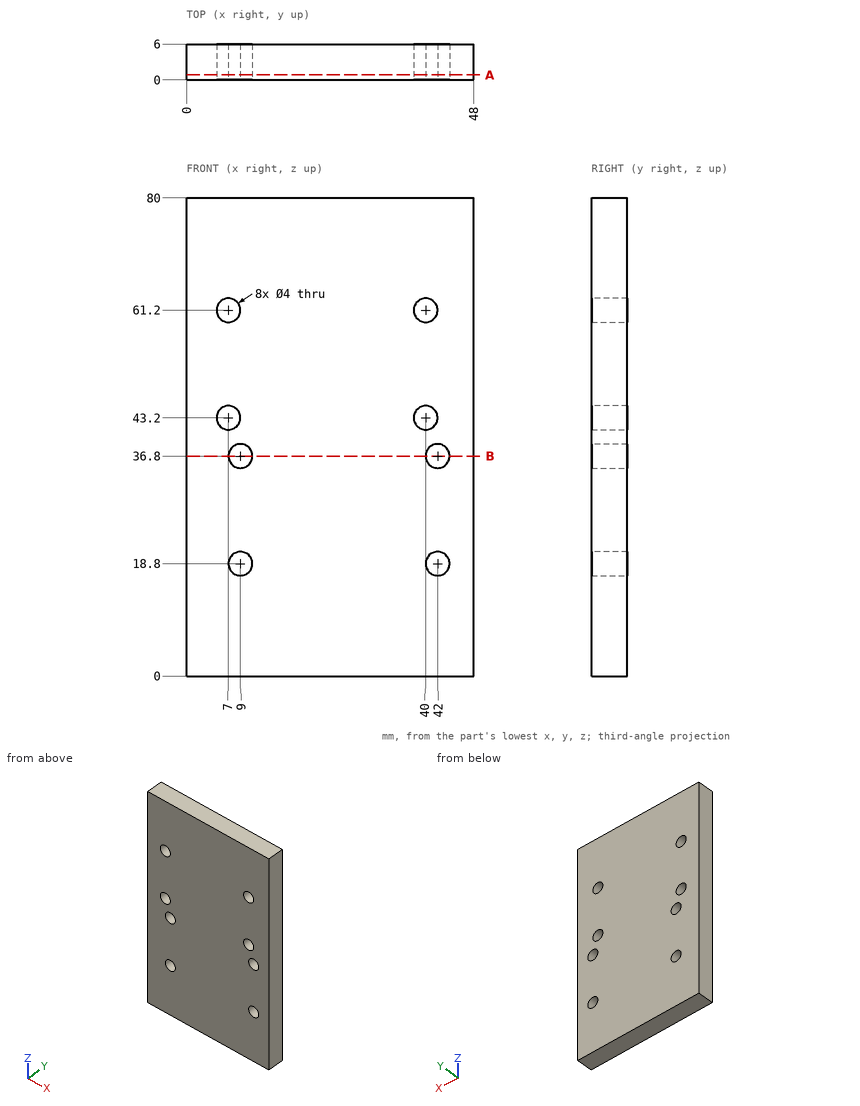
Can you work these out from the drawing? Everything is in mm from the part's minimum corner. Give positions to 0.01 mm unless a question says otherwise; leave off trailing zeros. Write each loop counter-clockwise with the first axis right and the second up, starting at its lowest first coordinate (ties: lowest second). Pieces come first, ordered by that corner, then holes. Notation, with made-up numbers: M 82,31.25 L 125,31.25 A13 cw 125,39.25 Z; hole C 53.25,11 d6. An arc over 180 degrees is marked long. Answer in a Markdown table with one row per item. Add a question column.
Item 1: Imagine slicing it at A-A, the plane y = 0.85. State how many separate pieces and enclosed holes the cut face has, plus the area to 3 significant figures.
Item 2: Please list where these lines run through material, in increasing order: L1, parallel to X at y = 4.3, z = 61.2; L2, parallel to X at y = 3.05, z = 18.8; L3, parallel to Z at x = 10.5, y = 4.7.
Item 3: Imagine slicing it at B-B, the plane z = 36.8. Write out the boundary of the cut face in (x, y).
Item 4: For pin 1 Ø3 at (x, z) = (7, 43.2) entering from +Y, with a flat end and sliding along its axis, tell me the tip position at first contact or that it passes through.
Evaluation:
| question | item | result |
|---|---|---|
| 1 | separate pieces | 1 |
| 1 | enclosed holes | 8 |
| 1 | area | 3,740 mm² |
| 2 | L1 | x = 0 to 5, 9 to 38, 42 to 48 |
| 2 | L2 | x = 0 to 7, 11 to 40, 44 to 48 |
| 2 | L3 | z = 0 to 17.48, 20.12 to 35.48, 38.12 to 80 |
| 3 | outline | M 0,0 L 7,0 L 7,6 L 0,6 Z; M 11,0 L 40,0 L 40,6 L 11,6 Z; M 44,0 L 48,0 L 48,6 L 44,6 Z |
| 4 | pin 1 | passes through |
